Work out the finished part from the listing and answer in its coordinate system (mm). A direction names the side the tool comes from. Give positions to 0.01 mm unless a question says otherwise; leave off trailing zeros. Loops run counter-clockwise (first coordinate to the right, second up) from the corner with the lowest first, then second, coordinate; pieces in that order, holes last. Notation, with made-up numbers: M 63.5,64 L 91.5,64 A29 ccw 91.5,90 Z; hole C 45,34.5 d9. An arc over 180 degrees is marked long. Use a Markdown table: item, result.
```python
from build123d import *

# Parameters (mm, degrees)
SKETCH_1_W                = 60
SKETCH_1_H                = 60
EXTRUDE_1_DEPTH           = 20
HOLE_WIZARD_1_D           = 5.5
HOLE_WIZARD_1_CBORE_D     = 10
HOLE_WIZARD_1_CBORE_DEPTH = 14
CHAMFER_1_SIZE            = 10
CHAMFER_2_SIZE            = 1
HOLE_WIZARD_M10_1_D       = 8.5
HOLE_WIZARD_M10_1_DEPTH   = 16.5
HOLE_WIZARD_M10_1_TIP     = 2.553657631


with BuildPart() as part:
    # 草图1 → 凸台-拉伸1 (new body)
    with BuildSketch(Plane.XY):
        Rectangle(SKETCH_1_W, SKETCH_1_H)
    extrude(amount=EXTRUDE_1_DEPTH)

    # 打孔尺寸(%根据)内六角圆柱头螺钉的类型1 (through all)
    with Locations(Plane(origin=(0, 0, 0), x_dir=(-1, 0, 0), z_dir=(0, 0, -1))):
        with Locations((-22.5, 15), (-22.5, -15), (-7.5, 15), (-7.5, -15), (22.5, -15), (7.5, 15), (7.5, -15), (22.5, 15)):
            CounterBoreHole(HOLE_WIZARD_1_D / 2, HOLE_WIZARD_1_CBORE_D / 2, HOLE_WIZARD_1_CBORE_DEPTH)

    # 倒角1
    chamfer_1_edges = [part.edges().sort_by_distance(p)[0] for p in [
        (30, -30, 10),
        (-30, -30, 10),
        (-30, 30, 10),
        (30, 30, 10),
    ]]
    chamfer(chamfer_1_edges, length=CHAMFER_1_SIZE)

    # 倒角2
    chamfer_2_edges = [part.edges().sort_by_distance(p)[0] for p in [
        (0, -30, 0),
        (0, -30, 20),
        (30, 0, 0),
        (-30, 0, 0),
        (0, 30, 0),
        (25, 25, 0),
        (25, -25, 0),
        (-25, 25, 0),
        (-25, -25, 0),
        (-30, 0, 20),
        (30, 0, 20),
        (0, 30, 20),
        (25, 25, 20),
        (25, -25, 20),
        (-25, 25, 20),
        (-25, -25, 20),
    ]]
    chamfer(chamfer_2_edges, length=CHAMFER_2_SIZE)

    # M10 螺纹孔1
    with Locations(Plane(origin=(0, 0, 0), x_dir=(-1, 0, 0), z_dir=(0, 0, -1))):
        with Locations((0, 0)):
            Hole(HOLE_WIZARD_M10_1_D / 2, depth=HOLE_WIZARD_M10_1_DEPTH)
            with Locations((0, 0, -(HOLE_WIZARD_M10_1_DEPTH + HOLE_WIZARD_M10_1_TIP / 2))):  # 118° drill point
                Cone(0, HOLE_WIZARD_M10_1_D / 2, HOLE_WIZARD_M10_1_TIP, mode=Mode.SUBTRACT)


solid = part.part
```
(1) Consider probe 1 along Y at (x, z) = (-7.5, 9.75); probe 2 along Y at (x, z) = (22.5, 9.25); probe 3 along Y at (x, z) = (0, 6.5). Determine where each line is inside the solid, lowest interval first. Write a range as [from, to].
Entries:
| item | result |
|---|---|
| probe 1 | y = [-30, -20], [-10, 10], [20, 30] |
| probe 2 | y = [-27.5, -20], [-10, 10], [20, 27.5] |
| probe 3 | y = [-30, -4.25], [4.25, 30] |
(2) A cutting plane is placed at B-B (x = 22). Write down the section's boundary in (y, z).
Entries:
| item | result |
|---|---|
| outline | M -28,1 L -26.59,0 L -19.97,0 L -19.97,14 L -17.7,14 L -17.7,20 L -26.59,20 L -28,19 Z; M -12.3,14 L -10.03,14 L -10.03,0 L 10.03,0 L 10.03,14 L 12.3,14 L 12.3,20 L -12.3,20 Z; M 17.7,14 L 19.97,14 L 19.97,0 L 26.59,0 L 28,1 L 28,19 L 26.59,20 L 17.7,20 Z |
(3) The mould has two halves that part along Z. Classify faces 3 (the cylindrical face through (10.12, -14.17, 17.04)), 4 (the flat face through (-24.71, 24.57, 19.51)), 5 (the flat face through (-25, 13, 14)): released by +Z, released by -Z, zero draft, split by the parting line, or undercut.
Entries:
| item | result |
|---|---|
| face 3 | zero draft |
| face 4 | released by +Z |
| face 5 | released by -Z |
(4) A cutting plane is placed at A-A (z = 3.5). Count the separate pieces of the cut face and the enclosed holes in it, and give its area (3 significant figures).
Entries:
| item | result |
|---|---|
| separate pieces | 1 |
| enclosed holes | 9 |
| area | 2,710 mm² |
(5) Given P1, Ø6.5, axis at x = -7.5, y = 15, coming from the -Z side, flat-ended and moving along its own axis, determine where the tip first touches the part or whether it passes through.
Entries:
| item | result |
|---|---|
| P1 | stops at z = 14 |
(6) Which of the six approach directions +Z, -Z, +X, -X, +Y, -Y give full straight-line access (tool end or side, diameter ignored) to faces 1 (the flat face through (-10, 13, 14)), 2 (the cylindrical face through (19.753, -14.879, 17.042))?
Entries:
| item | result |
|---|---|
| face 1 | -Z |
| face 2 | +Z, -Z |
(7) A cutting plane is placed at D-D (x = -7.5). Write down the section's boundary in (y, z).
Entries:
| item | result |
|---|---|
| outline | M -30,1 L -29,0 L -20,0 L -20,14 L -17.75,14 L -17.75,20 L -29,20 L -30,19 Z; M -12.25,14 L -10,14 L -10,0 L 10,0 L 10,14 L 12.25,14 L 12.25,20 L -12.25,20 Z; M 17.75,14 L 20,14 L 20,0 L 29,0 L 30,1 L 30,19 L 29,20 L 17.75,20 Z |
